from build123d import *

# Parameters (mm, degrees)
SKETCH_R          = 20.32
SKETCH_R_2        = 2.225
PAD_DEPTH         = 26.16
FILLET_R          = 0.5
SKETCH001_R       = 0.35
PAD001_DEPTH      = 13.08
PAD001_DEPTH_BACK = 3.5


with BuildPart() as fillet_body:
    # Sketch → Pad (new body)
    with BuildSketch(Plane.XY.offset(0.1)):
        with Locations((13.59, 0)):
            Circle(SKETCH_R)
        with Locations((13.59, 0)):
            Circle(SKETCH_R_2, mode=Mode.SUBTRACT)
    extrude(amount=PAD_DEPTH)

    # Fillet
    fillet_edges = [fillet_body.edges().sort_by_distance(p)[0] for p in [
        (11.365, 0, 26.26),
        (-6.73, 0, 26.26),
        (-6.73, 0, 0.1),
    ]]
    fillet(fillet_edges, radius=FILLET_R)


with BuildPart() as obj1:
    # Sketch001 → Pad001 (new body, two sides)
    with BuildSketch(Plane.XY.offset(0.5)) as pad001_sk:
        Circle(SKETCH001_R)
        with Locations((27.18, 0)):
            Circle(SKETCH001_R)
    extrude(amount=PAD001_DEPTH)
    extrude(pad001_sk.sketch, amount=-PAD001_DEPTH_BACK)

    # obj1: union Fillet body
    add(fillet_body.part)


solid = obj1.part
Input: part model. Units: mm. Frame: model coordinates. Coordinates: 2 decimals unless noted, no trailing zeros. Loops run counter-clockwise (first coordinate to the right, second up) from the corner with the lowest first, then second, coordinate; pieces in that order, holes last.
Q1. Cut plane B-B (z = 24.75). Output: boundary loops of the cut face in (x, y) (3 decimals).
Q2. Material intervals for line 1 (Y direction, x = 13.59, z = 9.25) (3 decimals); line 2 (Z direction, x = -4, y = -1); line 3 (X direction, y = -1.5, z = 21), sorted ascending.
Q3. Contact query for flat-ended pins moving along their axis: pin 1 (1 mm diameter, centred on y = 12.5, z = 13.5, fed in from +X); pin 2 (2 mm diameter, centred on y = -14, z = 3, fed in from +X); pin 3 (2 mm diameter, centred on y = -5.5, z = 19.5, fed in from -X); pin 4 (3.5 mm diameter, centred on x = 13.59, y = 0, fed in from -Z). Output: stop coordinate, or through.
Q4. Cut plane A-A (x = 13.59). Output: boundary loops of the cut face in (y, z) (3 decimals), then the cut area to 3 significant figures.
Working result:
1. outline: circle Ø40.64 at (13.59, 0); hole circle Ø4.45 at (13.59, 0)
2. line 1: y = -20.32 to -2.225, 2.225 to 20.32
2. line 2: z = 0.1 to 26.26
2. line 3: x = -6.67 to 11.95, 15.23 to 33.85
3. pin 1: stops at x = 29.99
3. pin 2: stops at x = 29.21
3. pin 3: stops at x = -6.23
3. pin 4: passes through
4. outline: (-20.32, 0.6) arc R0.5 ccw to (-19.82, 0.1) - (-2.225, 0.1) - (-2.225, 25.76) arc R0.5 ccw to (-2.725, 26.26) - (-19.82, 26.26) arc R0.5 ccw to (-20.32, 25.76) - close; (2.225, 0.1) - (19.82, 0.1) arc R0.5 ccw to (20.32, 0.6) - (20.32, 25.76) arc R0.5 ccw to (19.82, 26.26) - (2.725, 26.26) arc R0.5 ccw to (2.225, 25.76) - close
4. area: 946 mm2
